from build123d import *

# Parameters (mm, degrees)
F1_DEPTH = 2
F2_W     = 2.1478533745
F2_H     = 25.4813507199
F3_DEPTH = 2


with BuildPart() as f1:
    # F0 (on Top) → F1 (new body)
    with BuildSketch(Plane.XY):
        with BuildLine():
            Line((-50.4745617509, 15.1801089048), (-50.4745617509, -3.8698910952))
            Line((-50.4745617509, -3.8698910952), (-50.4745617509, -29.2698910952))
            Line((-50.4745617509, -29.2698910952), (-50.4745617509, -48.3198910952))
            Line((-50.4745617509, -48.3198910952), (-28.2495617509, -48.3198910952))
            Line((-28.2495617509, -48.3198910952), (-2.8495617509, -48.3198910952))
            Line((-2.8495617509, -48.3198910952), (19.3754382491, -48.3198910952))
            Line((19.3754382491, -48.3198910952), (19.3754382491, -29.2698910952))
            Line((19.3754382491, -29.2698910952), (19.3754382491, -3.8698910952))
            Line((19.3754382491, -3.8698910952), (19.3754382491, 15.1801089048))
            Line((19.3754382491, 15.1801089048), (19.3754382491, 55.8201089048))
            Line((19.3754382491, 55.8201089048), (-50.4745617509, 55.8201089048))
            Line((-50.4745617509, 55.8201089048), (-50.4745617509, 42.5905920565))
            add(Edge.make_bspline(
                [(-46.7963367701, 19.1511064768), (-45.3638130005, 21.1811384078), (-41.711839481, 26.3563570482), (-47.1621757409, 36.4539075513), (-50.4745617509, 42.5905920565)],
                knots=[0, 0, 0, 0, 0.3922601785, 1, 1, 1, 1], degree=3))
            Line((-46.7963367701, 19.1511064768), (-50.4745617509, 22.4870592356))
            Line((-50.4745617509, 22.4870592356), (-50.4745617509, 15.1801089048))
        make_face()
    extrude(amount=F1_DEPTH)

    # F2 (on Top) → F3 (join)
    with BuildSketch(Plane.XY):
        with Locations((18.1335583329, -16.6092142463)):
            Rectangle(F2_W, F2_H)
    extrude(amount=-F3_DEPTH)


solid = f1.part
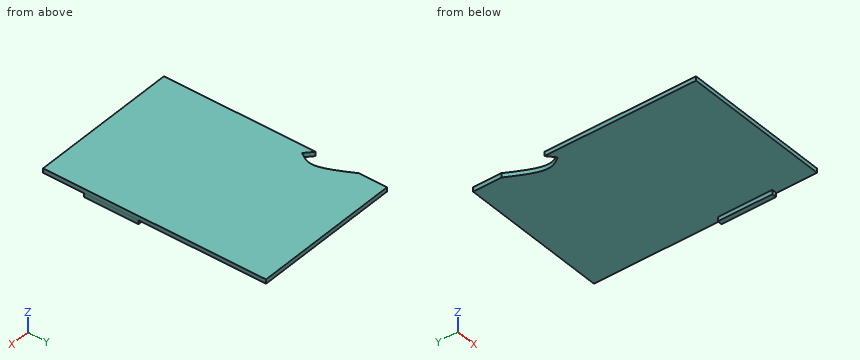
Geometry check sheet. Reference: the model listing, model coordinates, mm. Give positions to 0.01 mm unless a question says otherwise; leave off trailing zeros. Order: outer loops, then holes, each group sorted by start corner. A loop starts at its lowest first (then second) coordinate and runs counter-clockwise, first axis right, second up. Notation, with made-up numbers: (-4.5, 61) - (11.5, 61) arc R16 ccw to (11.5, 75) - close; hole circle Ø4 at (86.5, 74). An arc over 180 degrees is marked (long way). Use one line per item in the form item = value.
1) Sectioned sample at B-B (x = -22). Record the boundary of the cut face in (y, z).
Working result:
outline = (-48.32, 0) - (55.82, 0) - (55.82, 2) - (-48.32, 2) - close
2) Depth check by flat-ended pin: pin 1 Ø2 at (x, y) = (3.5, -33.5) entering from -Z; pin 2 Ø1 at (x, z) = (18, -1) entering from -Y; pin 3 Ø1.6 at (y, z) = (-10.5, -1.5) entering from -X; pin 4 Ø1 at (y, z) = (34.5, -1) entering from -X. Enter the tip coordinate at first touch or a pass-through.
Working result:
pin_1 = 0
pin_2 = -29.35
pin_3 = 17.06
pin_4 = through
3) Sectioned sample at A-A (y = -25.5). Record the boundary of the cut face in (x, z), and give its area (3 significant figures).
Working result:
outline = (-50.47, 0) - (17.06, 0) - (17.06, -2) - (19.21, -2) - (19.21, 0) - (19.38, 0) - (19.38, 2) - (-50.47, 2) - close
area = 144 mm^2
4) Material ranges on probe 1 along Z at (x, y) = (-43, 10); probe 2 along X at (y, z) = (-17.5, -0.75); probe 3 along X at (y, z) = (38.5, 0.15), recorded low to high. Write a range as from..to.
Working result:
probe_1 = 0..2
probe_2 = 17.06..19.21
probe_3 = -48.29..19.38
5) Sectioned sample at C-C (z = -0.8). Record the boundary of the cut face in (x, y), and give its area (3 significant figures).
Working result:
outline = (17.06, -29.35) - (19.21, -29.35) - (19.21, -3.87) - (17.06, -3.87) - close
area = 54.7 mm^2
